Input: part model. Units: mm. Frame: model coordinates. Face numbers are marked on the shaded views. Round coordinates to 2 decimals unless told otherwise and drop trailing zeros. Loops run counter-clockwise (first coordinate to the right, second up) from the corner with the lowest first, then second, coordinate; pieces in that order, holes last. Notation, with made-up numbers: (49.25, 76.5) - (104.25, 76.5) arc R25 cw to (104.25, 107.5) - close; hole circle Ø8 at (20, 34). An arc over 180 degrees is marked (long way). Write each question's results on one line, items separated by ' | '.
from build123d import *

# Parameters (mm, degrees)
F0_W     = 50.8
F0_H     = 203.2
F1_DEPTH = 83.865166
F2_R     = 21.886059
F3_DEPTH = 50.801


with BuildPart() as f1:
    # F0 (on Right) → F1 (new body)
    with BuildSketch(Plane.YZ):
        with Locations((-69.854085, 10.577654)):
            Rectangle(F0_W, F0_H)
    extrude(amount=F1_DEPTH)

    # F2 (on face) → F3 (cut, through all)
    with BuildSketch(Plane.XZ.offset(95.254085)):
        with Locations((48.370779, 0)):
            Circle(F2_R)
    extrude(amount=-F3_DEPTH, mode=Mode.SUBTRACT)


solid = f1.part
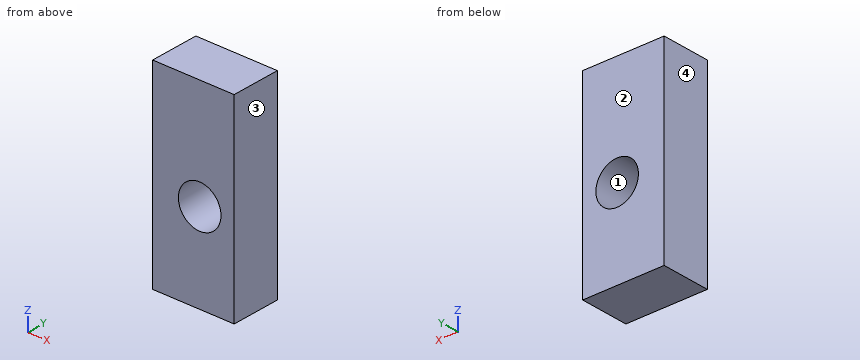
1. Mould query, pull axis X, two halves, no side actions, for the marked faces 1, 2, 3 and 4. Classes: pulls with the +X half, pulls with the -X half, needs draft (parallel to the pull), parting line crosses it, or undercut.
Answer:
face 1: undercut | face 2: needs draft | face 3: pulls with the +X half | face 4: pulls with the -X half
2. Section query C-C, the plane y = -61.5. Output: boundary loops of the cut face in (x, z), plus the area to 3 significant figures.
Answer:
outline: (0, -91.02) - (83.87, -91.02) - (83.87, 112.18) - (0, 112.18) - close; hole circle Ø43.77 at (48.37, 0) | area: 15,500 mm^2
3. Section query A-A, the plane z = 0. Output: boundary loops of the cut face in (x, y), plus the area to 3 significant figures.
Answer:
outline: (0, -95.25) - (26.48, -95.25) - (26.48, -44.45) - (0, -44.45) - close; (70.26, -95.25) - (83.87, -95.25) - (83.87, -44.45) - (70.26, -44.45) - close | area: 2,040 mm^2
4. Section query B-B, the plane x = 32. Output: boundary loops of the cut face in (y, z), plus the area to 3 significant figures.
Answer:
outline: (-95.25, -91.02) - (-44.45, -91.02) - (-44.45, -14.53) - (-95.25, -14.53) - close; (-95.25, 14.53) - (-44.45, 14.53) - (-44.45, 112.18) - (-95.25, 112.18) - close | area: 8,850 mm^2
5. Line query: line 1 (Z direction, x = 42, y = -53); line 2 (X direction, y = -67, z = 1); line 3 (Z direction, x = 61, y = -70.5). Output: solid intervals per line, ascending. Write a range as [from, to].
Answer:
line 1: [-91.02, -20.94], [20.94, 112.18] | line 2: [0, 26.51], [70.23, 83.87] | line 3: [-91.02, -17.87], [17.87, 112.18]
